Could you check a few things on this model? Use its own coordinates, in mm. Face numbers are marked on the shaded views. A direction names the side the tool comes from. Coordinates: 2 decimals unless noted, no trailing zeros. Order: outer loops, then holes, each group sorted by start corner. A loop starts at its lowest first (then second) coordinate and runs counter-clockwise, first axis right, second up. Notation, with made-up numbers: (-5.75, 64.25) -> (5.25, 64.25) arc R26 cw to (5.25, 83.25) -> close; hole circle Ø11 at (-33.5, 20.5). An arc over 180 degrees is marked (long way). Use a Markdown table: item, result. Add a question column.
1) If we section it at A-A (x = 6): Write out the boundary of the cut face in (y, z), plus the area to 3 significant figures.
2) If we section it at B-B (z = 7): Write out the boundary of the cut face in (x, y), plus the area to 3 significant figures.
3) If I drill on L1, parallel to Z at x = -40.5, y = -17.25; L2, parallel to Y at x = -7.5, z = -29; L3, parallel to X at y = -23, z = -44, over which ranges is the centre line in solid material (lowest first)? Write a range as [from, to].
4) Thinking about a two-plate mould opening in Z: for the marked faces 1, 2 and 3, which applies, +Z half, -Z half, draft (parallel to the pull), parting line (faces both ways), or undercut?
5) Which directions (+Z, -Z, +X, -X, +Y, -Y) give clear straight access to the entire face, cutting with the end or side of a thin tool? Please do the marked faces 4 and 5.
6) If we section it at C-C (y = -23.5): Write out the boundary of the cut face in (x, z), plus the area to 3 significant figures.
7) Will these pins go through, and if not, where does the flat tip stop? pin 1 Ø3 at (y, z) = (-9, -50.5) entering from -X; pin 2 Ø23 at (x, z) = (-21.5, 21.5) entering from +Y; pin 3 Ø5 at (x, y) = (-27.5, -19) entering from -Z.
Autodesk Inventor part; units mm, degrees
ref_plane "Work Plane1" through (0, 2.54, 0) normal (0, 1, 0) x (-1, 0, 0)
ref_plane "YZ Plane" through (0, 0, 0) normal (1, 0, 0) x (0, 1, 0)
ref_plane "XY Plane" through (0, 0, 0) normal (0, 0, 1) x (1, 0, 0)
sketch "Sketch1" plane through (0, 0, 0) normal (0, 1, 0) x (-1, 0, 0)
  line L0 (60.96, -81.28) -> (-40.64, -81.28)
  line L1 (-40.64, -81.28) -> (-40.64, 71.12)
  line L2 (-40.64, 71.12) -> (60.96, 71.12)
  line L3 (60.96, 71.12) -> (60.96, -81.28)
  point P0 (0, 0)
  dimension "d0" = 152.4
  dimension "d1" = 101.6
extrude "Extrusion1" add sketch "Sketch1" along normal blind 2.54
sketch "Sketch2" plane through (0, 0, 0) normal (0, 1, 0) x (-1, 0, 0)
  line L0 (48.26, 57.7273) -> (-27.94, 57.7273)
  line L1 (-27.94, 57.7273) -> (-27.94, -69.2727)
  line L2 (-27.94, -69.2727) -> (48.26, -69.2727)
  line L3 (48.26, -69.2727) -> (48.26, 57.7273)
  line L4 (60.96, -81.28) -> (60.96, 71.12)
  line L5 (-40.64, 71.12) -> (-40.64, -81.28)
  point P0 (0, 0)
  dimension "d4" = 127
  dimension "d5" = 76.2
  dimension "d11" = 12.7
extrude "Extrusion2" add sketch "Sketch2" against normal blind 25.4
ref_plane "Work Plane1" through (0, 2.54, 0) normal (0, 1, 0) x (-1, 0, 0)
sketch "Sketch3" plane through (0, 2.54, 0) normal (0, 1, 0) x (-1, 0, 0)
  line L0 (48.26, 57.7273) -> (48.26, -69.2727)
  line L1 (-27.94, -69.2727) -> (-27.94, 57.7273)
  line L2 (48.26, 57.7273) -> (-27.94, 57.7273)
  line L3 (-27.94, 57.7273) -> (-27.94, -69.2727)
  line L4 (-27.94, -69.2727) -> (48.26, -69.2727)
  line L5 (48.26, -69.2727) -> (48.26, 57.7273)
  point P0 (0, 0)
extrude "Extrusion3" cut sketch "Sketch3" against normal blind 1.27
properties part number "Computer"
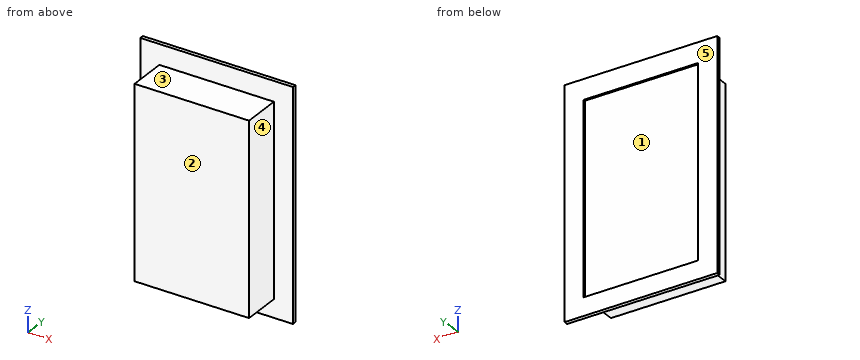
Answer sheet:
| question | item | result |
|---|---|---|
| 1 | outline | (-25.4, -69.27) -> (0, -69.27) -> (0, -81.28) -> (2.54, -81.28) -> (2.54, -69.27) -> (1.27, -69.27) -> (1.27, 57.73) -> (2.54, 57.73) -> (2.54, 71.12) -> (0, 71.12) -> (0, 57.73) -> (-25.4, 57.73) -> close |
| 1 | area | 3,450 mm2 |
| 2 | outline | (-60.96, 0) -> (-48.26, 0) -> (-48.26, -25.4) -> (27.94, -25.4) -> (27.94, 0) -> (40.64, 0) -> (40.64, 2.54) -> (27.94, 2.54) -> (27.94, 1.27) -> (-48.26, 1.27) -> (-48.26, 2.54) -> (-60.96, 2.54) -> close |
| 2 | area | 2,100 mm2 |
| 3 | L1 | [-69.27, 57.73] |
| 3 | L2 | [-25.4, 1.27] |
| 3 | L3 | [-48.26, 27.94] |
| 4 | face 1 | undercut |
| 4 | face 2 | draft |
| 4 | face 3 | +Z half |
| 5 | face 4 | +Z, -Z, +X, -Y |
| 5 | face 5 | +Z, -Z, +X, -X, +Y |
| 6 | outline | (-48.26, -69.27) -> (27.94, -69.27) -> (27.94, 57.73) -> (-48.26, 57.73) -> close |
| 6 | area | 9,680 mm2 |
| 7 | pin 1 | x = -48.26 |
| 7 | pin 2 | y = 1.27 |
| 7 | pin 3 | z = -69.27 |
